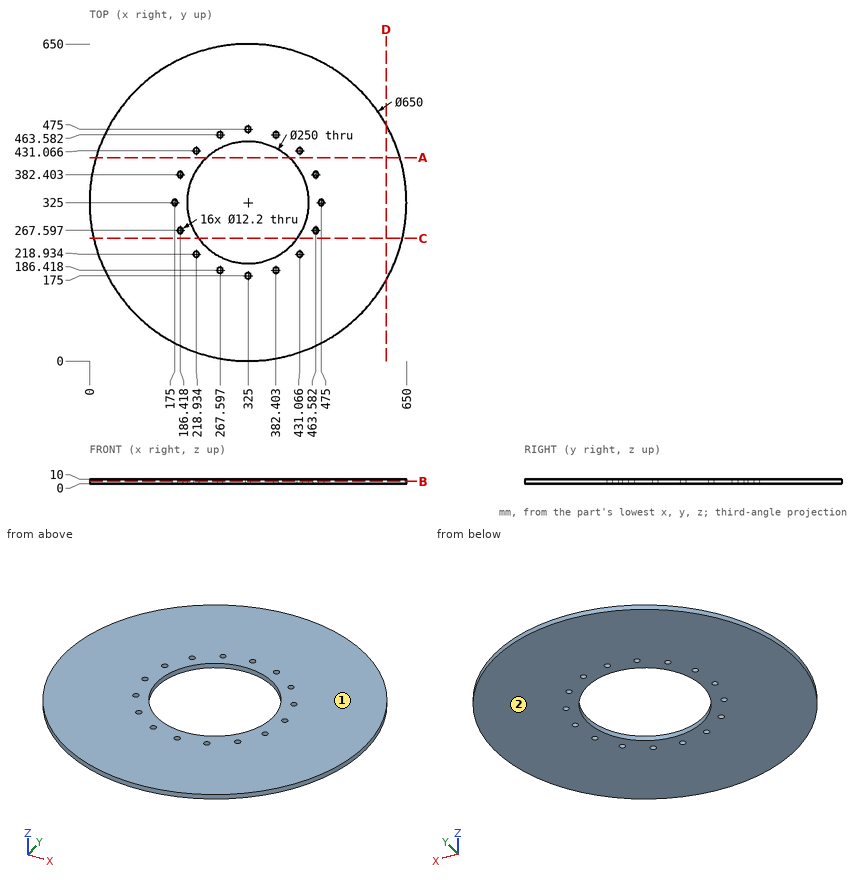
Could you check a few things on this drawing? It's one solid part, dimensions in mm from its lowest x, y, z. Round coordinates to 2 decimals unless told otherwise and drop trailing zeros. Loops run counter-clockwise (first coordinate to the right, second up) from the corner with the lowest first, then second, coordinate; pieces in that order, holes last. Notation, with made-up numbers: (10, 13) -> (21, 13) arc R35 cw to (21, 45) -> close; hole circle Ø11 at (-22.5, 3.25). An arc over 180 degrees is marked (long way). One line per item, written item: value. Start each with the question number.
1. If we mould it in two halves opening along Z, with no side actions, what happens to the marked faces 1 and 2? For each: pulls with the +Z half, pulls with the -Z half, needs draft (parallel to the pull), parting line crosses it, or undercut.
2. If we section it at A-A, the plane y = 417: Write out the boundary of the cut face in (x, z), then the cut area to 3 significant figures.
3. If we section it at C-C, the plane y = 251.5: Write out the boundary of the cut face in (x, z), then the cut area to 3 significant figures.
4. If we section it at B-B, the plane z = 5.25: Give the number of separate pieces and of enclosed holes in the cut face, then the cut area to 3 significant figures.
5. For pin 1 (7.5 mm diameter, centred on x = 382.4, y = 463.58, fed in from -Z); pin 2 (6 mm diameter, centred on y = 283, z = 1, fed in from -X); pin 3 (4 mm diameter, centred on x = 554, z = 5.5, fed in from +Y) (1 decimal); pin 4 (2 mm diameter, centred on x = 196, z = 2, fed in from -Y), each with a flat end and sliding along its axis, tell me the tip position at first contact or that it passes through.
6. If I drill on probe 1 along Y at (x, z) = (325, 7.75); probe 2 along Y at (x, z) = (465, 9.75) (1 decimal); probe 3 along X at (y, z) = (434, 9) (1 decimal), over which ranges is the centre line in solid material (lowest first)?
7. If we section it at D-D, the plane x = 608: Write out the boundary of the cut face in (y, z), then the cut area to 3 significant figures.
Calculated:
1. face 1: pulls with the +Z half
1. face 2: pulls with the -Z half
2. outline: (13.29, 0) -> (240.38, 0) -> (240.38, 10) -> (13.29, 10) -> close; (409.62, 0) -> (636.71, 0) -> (636.71, 10) -> (409.62, 10) -> close
2. area: 4,540 mm²
3. outline: (8.42, 0) -> (223.89, 0) -> (223.89, 10) -> (8.42, 10) -> close; (426.11, 0) -> (641.58, 0) -> (641.58, 10) -> (426.11, 10) -> close
3. area: 4,310 mm²
4. separate pieces: 1
4. enclosed holes: 17
4. area: 281,000 mm²
5. pin 1: passes through
5. pin 2: stops at x = 2.35
5. pin 3: stops at y = 557.6
5. pin 4: stops at y = 26.27
6. probe 1: y = 0 to 168.9, 181.1 to 200, 450 to 468.9, 481.1 to 650
6. probe 2: y = 31.7 to 261.7, 273.5 to 376.5, 388.3 to 618.3
6. probe 3: x = 18.8 to 213.6, 224.3 to 263.8, 386.2 to 425.7, 436.4 to 631.2
7. outline: (165.2, 0) -> (484.8, 0) -> (484.8, 10) -> (165.2, 10) -> close
7. area: 3,200 mm²
